The model under review builds one solid part; all positions refer to its coordinate system, in mm. A direction names the side the tool comes from. Coordinates: 2 decimals unless noted, no trailing zeros. Write each loop counter-clockwise with the first axis right and the second up, starting at its lowest first coordinate (ties: lowest second). Pieces come first, ordered by that corner, then holes. Notation, with made-up numbers: (77.5, 55.5) -> (107.5, 55.5) arc R9 ccw to (107.5, 62.5) -> close; hole circle Ø7 at (11.5, 39.25). An arc over 180 degrees is marked (long way). Write each question's results on one line, items separated by ' | '.
```python
from build123d import *

# Parameters (mm, degrees)
SKETCH6_R                                = 66.04
BOSS_EXTRUDE1_DEPTH                      = 2.54
PIPE_TAP_DRILL_FOR_1_4_TAP_RELIEF_VALV_D = 11.1252
PIPE_TAP_DRILL_FOR_1_4_TAP_VENT_VALVE_D  = 11.1252


with BuildPart() as part:
    # Sketch1 → Revolve1 (revolve)
    with BuildSketch(Plane.XY, mode=Mode.PRIVATE) as revolve1_sk:
        Polygon((0, 0), (72.898, 0), (72.898, 2.4638), (69.977, 2.4638), (69.977, 7.4422), (72.898, 7.4422), (72.898, 9.906), (66.548, 9.906), (66.548, 6.35), (0, 6.35), align=None)
    revolve(revolve1_sk.sketch.rotate(Axis((0, 48.192213231, 0), (0, -1, 0)), 180), axis=Axis((0, 48.192213231, 0), (0, -1, 0)))

    # Sketch6 → Boss-Extrude1 (add)
    with BuildSketch(Plane.XZ):
        Circle(SKETCH6_R)
    extrude(amount=BOSS_EXTRUDE1_DEPTH)

    # Pipe Tap Drill for 1/4 Tap - Relief Valve (through all)
    with Locations(Plane(origin=(0, -2.54, 0), x_dir=(-1, 0, 0), z_dir=(0, -1, 0))):
        with Locations((0, 44.958)):
            Hole(PIPE_TAP_DRILL_FOR_1_4_TAP_RELIEF_VALV_D / 2)

    # Pipe Tap Drill for 1/4 Tap - Vent Valve (through all)
    with Locations(Plane(origin=(0, -2.54, 0), x_dir=(-1, 0, 0), z_dir=(0, -1, 0))):
        with Locations((0, -44.958)):
            Hole(PIPE_TAP_DRILL_FOR_1_4_TAP_VENT_VALVE_D / 2)


solid = part.part
```
Q1. Clearance check with flat-ended pins moving along their axes: P1, Ø1.5, axis at y = 0.5, z = -40, coming from the +X side; P2, Ø6, axis at x = -8.5, y = 7.5, coming from the -Z side; P3, Ø1, axis at y = 1, z = -15, coming from the +X side; P4, Ø10, axis at x = 0, z = -44.958, coming from the +Y side. State where each tip first meets the part, or that it passes through.
Solution:
P1: x = 61.43 | P2: z = -72.69 | P3: x = 71.44 | P4: through
Q2. For line 1 (Z direction, x = 0, y = 3); line 2 (Z direction, x = 0, y = 9); line 3 (Y direction, x = -33.5, z = 62.5), list the stretches that pass through material, from the lowest coordinate up. Write a range as from..to.
Solution:
line 1: -69.98..-50.52, -39.4..39.4, 50.52..69.98 | line 2: -72.9..-66.55, 66.55..72.9 | line 3: 0..2.46, 7.44..9.91
Q3. Machinability: for faces 1 (the flat face through (1, 6.35, -1)), 2 (the flat face through (-38.1, 0, -54.3)), 3 (the cylindrical face through (-66.746, 4.988, -21.019)), which of the approach directions +Z, -Z, +X, -X, +Y, -Y give a long, thin tool a straight path to every point of the face, cutting with its end or side? Answer none if there is none.
Solution:
face 1: +Y | face 2: -Y | face 3: none
Q4. Add section B-B (z = 0). Write out the cut boundary in (x, y).
Solution:
outline: (-72.9, 0) -> (-66.04, 0) -> (-66.04, -2.54) -> (66.04, -2.54) -> (66.04, 0) -> (72.9, 0) -> (72.9, 2.46) -> (69.98, 2.46) -> (69.98, 7.44) -> (72.9, 7.44) -> (72.9, 9.91) -> (66.55, 9.91) -> (66.55, 6.35) -> (-66.55, 6.35) -> (-66.55, 9.91) -> (-72.9, 9.91) -> (-72.9, 7.44) -> (-69.98, 7.44) -> (-69.98, 2.46) -> (-72.9, 2.46) -> close
Q5. Draft analysis for pull direction X (two halves, no side actions). For faces 4 (the cylindrical face through (-1.206, 1.967, 50.388)), 5 (the cylindrical face through (15.803, 8.691, 71.165)), 6 (the flat face through (-65, 7.442, -27)), state which applies: pulls with the +X half, pulls with the -X half, needs draft (parallel to the pull), parting line crosses it, or undercut.
Solution:
face 4: undercut | face 5: parting line crosses it | face 6: needs draft
Q6. Add section A-A (x = 0). Write out the cut boundary in (y, z), plus the area to 3 significant figures.
Solution:
outline: (-2.54, -66.04) -> (0, -66.04) -> (0, -72.9) -> (2.46, -72.9) -> (2.46, -69.98) -> (7.44, -69.98) -> (7.44, -72.9) -> (9.91, -72.9) -> (9.91, -66.55) -> (6.35, -66.55) -> (6.35, -50.52) -> (-2.54, -50.52) -> close; (-2.54, -39.4) -> (6.35, -39.4) -> (6.35, 39.4) -> (-2.54, 39.4) -> close; (-2.54, 50.52) -> (6.35, 50.52) -> (6.35, 66.55) -> (9.91, 66.55) -> (9.91, 72.9) -> (7.44, 72.9) -> (7.44, 69.98) -> (2.46, 69.98) -> (2.46, 72.9) -> (0, 72.9) -> (0, 66.04) -> (-2.54, 66.04) -> close | area: 1,080 mm²
Q7. Add section C-C (x = 23.5). Write out the cut boundary in (y, z), plus the area to 3 significant figures.
Solution:
outline: (-2.54, -61.72) -> (0, -61.72) -> (0, -69.01) -> (2.46, -69.01) -> (2.46, -65.91) -> (7.44, -65.91) -> (7.44, -69.01) -> (9.91, -69.01) -> (9.91, -62.26) -> (6.35, -62.26) -> (6.35, 62.26) -> (9.91, 62.26) -> (9.91, 69.01) -> (7.44, 69.01) -> (7.44, 65.91) -> (2.46, 65.91) -> (2.46, 69.01) -> (0, 69.01) -> (0, 61.72) -> (-2.54, 61.72) -> close | area: 1,210 mm²
